Autodesk Inventor part; units mm, degrees
ref_plane "YZ Plane" through (0, 0, 0) normal (1, 0, 0) x (0, 1, 0)
ref_plane "XZ Plane" through (0, 0, 0) normal (0, 1, 0) x (-1, 0, 0)
ref_plane "XY Plane" through (0, 0, 0) normal (0, 0, 1) x (1, 0, 0)
sketch "Sketch1" plane through (0, 0, 0) normal (0, 0, 1) x (1, 0, 0)
  line L0 (-12.1708, 16.0073) -> (13.2292, 16.0073)
  line L1 (13.2292, 16.0073) -> (13.2292, -34.7927)
  line L2 (13.2292, -34.7927) -> (-12.1708, -34.7927)
  line L3 (-12.1708, -34.7927) -> (-12.1708, 16.0073)
  line L4 (11.9592, 14.7373) -> (-10.9008, 14.7373)
  line L5 (-10.9008, 14.7373) -> (-10.9008, -33.5227)
  line L6 (-10.9008, -33.5227) -> (11.9592, -33.5227)
  line L7 (11.9592, -33.5227) -> (11.9592, 14.7373)
  point P0 (0, 0)
  dimension "d0" = 25.4
  dimension "d1" = 50.8
  dimension "d2" = 1.27
extrude "Extrusion1" add sketch "Sketch1" along normal blind 533.4
sketch "Sketch2" plane through (-12.1708, 16.0073, 0) normal (0, 1, 0) x (1, 0, 0)
  circle A0 centre (12.7, -12.7) radius 1.7272
  line L0 (25.4, 0) -> (0, 0)
  line L1 (0, 0) -> (0, -533.4)
  point P0 (12.1708, 0)
  dimension "d5" = 3.4544
  dimension "d6" = 12.7
  dimension "d7" = 12.7
extrude "Extrusion2" cut sketch "Sketch2" against normal through all
pattern_linear "Rectangular Pattern1" count 21 spacing 25.4 along (0, 0, 1) of "Extrusion2"
equation "\"d3\" = d13"
equation "\"d13\" = 533.4"
properties part number "VerseFrame 21in"
Here's how the part is built. I have some questions about the finished solid (model axes, mm). A direction names the side the tool comes from. Give positions to 0.01 mm unless a question says otherwise; leave off trailing zeros. Order: outer loops, then holes, each group sorted by start corner. A loop starts at its lowest first (then second) coordinate and runs counter-clockwise, first axis right, second up. Notation, with made-up numbers: (-16, 66.25) -> (12, 66.25) arc R33 cw to (12, 96.25) -> close; hole circle Ø10 at (25, -27.5). An arc over 180 degrees is marked (long way). One line per item, written item: value. Start each with the question number.
1. Imagine slicing it at A-A, the plane y = -0.5. List the corners of the cut face in (x, z) for me.
2. Will this pin go through, and if not, where does the flat tip stop? pin 1 Ø2 at (x, z) = (0.53, 88.9) entering from +Y.
3. We'd pull the mould along X, two halves only. Please class faces 1 (the face through (-12, -9, 0)), 2 (the face through (-12.171, -10, 263)), 3 (the face through (0, -33.523, 263)): released by +X, released by -X, zero draft, split by the parting line, or undercut.
4. I need wall thicknesses on probe 1 along Y at (x, z) = (3, 466.5); probe 2 along X at (y, z) = (-16.5, 322); probe 3 along X at (y, z) = (-33.8, 342.9). Which ranges of each line are inside material? Lowest first, please. Write a range as from..to.
5. For faces 4 (the face through (0, 16.007, 263)), 5 (the face through (11.959, -10, 263)), which set-ups out of +Z, -Z, +X, -X, +Y, -Y let a thin tool reach every point of the face, with its end or its side?
Values follow:
1. outline: (-12.17, 0) -> (-10.9, 0) -> (-10.9, 533.4) -> (-12.17, 533.4) -> close; (11.96, 0) -> (13.23, 0) -> (13.23, 533.4) -> (11.96, 533.4) -> close
2. pin 1: passes through
3. face 1: zero draft
3. face 2: released by -X
3. face 3: undercut
4. probe 1: y = -34.79..-33.52, 14.74..16.01
4. probe 2: x = -12.17..-10.9, 11.96..13.23
4. probe 3: x = -12.17..-1.2, 2.26..13.23
5. face 4: +Z, -Z, +X, -X, +Y
5. face 5: +Z, -Z
